```python
from build123d import *

# Parameters (mm, degrees)
SKETCH005_R       = 41.5
SKETCH005_R_2     = 12.75
PAD001_DEPTH      = 16.5
CYLINDER003_R     = 16
CYLINDER003_DEPTH = 25.2
CYLINDER008_R     = 4
CYLINDER008_DEPTH = 25
CYLINDER009_R     = 4
CYLINDER009_DEPTH = 25
POCKET_START      = -1.25
SKETCH084_R       = 48
SKETCH084_R_2     = 40
POCKET_DEPTH      = 14


with BuildPart() as part:
    # Sketch005 → Pad001 (new body)
    with BuildSketch(Plane.XY):
        with Locations((0, -21.25)):
            Circle(SKETCH005_R)
        Circle(SKETCH005_R_2, mode=Mode.SUBTRACT)
        with BuildLine():
            ThreePointArc((-31.480397, -26.993223), (-24.225688, -42.15732), (-10.285714, -51.551882))
            ThreePointArc((-10.285714, -51.551882), (-6.670071, -51.015521), (-5, -47.764147))
            Line((-5, -27.568098), (-5, -47.764147))
            ThreePointArc((-5, -27.568098), (-5.762291, -25.219217), (-7.758621, -23.765601))
            ThreePointArc((-16.637158, -18.660251), (-12.462129, -21.672456), (-7.758621, -23.765601))
            ThreePointArc((-16.637158, -18.660251), (-27.032318, -17.53007), (-31.480397, -26.993223))
        make_face(mode=Mode.SUBTRACT)
        with BuildLine():
            ThreePointArc((10.285714, -51.551882), (24.225688, -42.15732), (31.480397, -26.993223))
            ThreePointArc((31.480397, -26.993223), (27.032318, -17.53007), (16.637158, -18.660251))
            ThreePointArc((7.758621, -23.765601), (12.462129, -21.672456), (16.637158, -18.660251))
            ThreePointArc((7.758621, -23.765601), (5.762291, -25.219217), (5, -27.568098))
            Line((5, -27.568098), (5, -47.764147))
            ThreePointArc((5, -47.764147), (6.670071, -51.015521), (10.285714, -51.551882))
        make_face(mode=Mode.SUBTRACT)
    extrude(amount=-PAD001_DEPTH)

    # Cylinder003 → Cylinder003 (cut)
    with BuildSketch(Plane.XY.offset(-12.5)):
        Circle(CYLINDER003_R)
    extrude(amount=CYLINDER003_DEPTH, mode=Mode.SUBTRACT)

    # Cylinder008 → Cylinder008 (cut)
    with BuildSketch(Plane(origin=(23, 0, -13), x_dir=(1, 0, 0), z_dir=(0, 0, 1))):
        Circle(CYLINDER008_R)
    extrude(amount=CYLINDER008_DEPTH, mode=Mode.SUBTRACT)

    # Cylinder009 → Cylinder009 (cut)
    with BuildSketch(Plane(origin=(-23, 0, -13), x_dir=(1, 0, 0), z_dir=(0, 0, 1))):
        Circle(CYLINDER009_R)
    extrude(amount=CYLINDER009_DEPTH, mode=Mode.SUBTRACT)

    # Sketch084 → Pocket (cut)
    with BuildSketch(Plane.XY.offset(POCKET_START)):
        with Locations((0, -21.25)):
            Circle(SKETCH084_R)
        with Locations((0, -21.25)):
            Circle(SKETCH084_R_2, mode=Mode.SUBTRACT)
    extrude(amount=-POCKET_DEPTH, mode=Mode.SUBTRACT)


solid = part.part
```
The model under review builds one solid part; all positions refer to its coordinate system, in mm. A direction names the side the tool comes from. Round coordinates to 2 decimals unless told otherwise and drop trailing zeros. Loops run counter-clockwise (first coordinate to the right, second up) from the corner with the lowest first, then second, coordinate; pieces in that order, holes last. Notation, with made-up numbers: M 1,60.5 L 23,60.5 A21 ccw 23,69.5 Z; hole C 9,11 d7. An arc over 180 degrees is marked long. Put each result on its own line as item: value.
Q1. Consider section C-C, the plane y = 0. Give the boundary of the cut face in (x, z).
Result set:
outline: M -35.65,-16.5 L -12.75,-16.5 L -12.75,-12.5 L -16,-12.5 L -16,0 L -19,0 L -19,-13 L -27,-13 L -27,0 L -35.65,0 L -35.65,-1.25 L -33.89,-1.25 L -33.89,-15.25 L -35.65,-15.25 Z; M 12.75,-16.5 L 35.65,-16.5 L 35.65,-15.25 L 33.89,-15.25 L 33.89,-1.25 L 35.65,-1.25 L 35.65,0 L 27,0 L 27,-13 L 19,-13 L 19,0 L 16,0 L 16,-12.5 L 12.75,-12.5 Z
Q2. Consider section D-D, the plane y = -21.25. Give the boundary of the cut face in (x, z).
Result set:
outline: M -41.5,-16.5 L -30.62,-16.5 L -30.62,0 L -41.5,0 L -41.5,-1.25 L -40,-1.25 L -40,-15.25 L -41.5,-15.25 Z; M -13.17,-16.5 L 13.17,-16.5 L 13.17,0 L -13.17,0 Z; M 30.62,-16.5 L 41.5,-16.5 L 41.5,-15.25 L 40,-15.25 L 40,-1.25 L 41.5,-1.25 L 41.5,0 L 30.62,0 Z
Q3. Mouldability with a two-part tool opening along Y and no side actions: class faces 1 (the flat face through (5, -38, -8)), 2 (the cylindrical face through (-30.587, 6.798, -0.616)), 3 (the flat face through (-22, 13, -1.25)) as released by +Y, released by -Y, zero draft, split by the parting line, or undercut.
Result set:
face 1: undercut
face 2: split by the parting line
face 3: zero draft
Q4. Machinability: for faces 4 (the cylindrical face through (12.4, -21.71, -8.13)), 5 (the flat face through (23, 0, -13)), 6 (the flat face through (-22, 13, -15.25)), which of the approach directions +Z, -Z, +X, -X, +Y, -Y give a long, thin tool a straight path to every point of the face, cutting with its end or side? Answer none if there is none.
Result set:
face 4: +Z, -Z
face 5: +Z
face 6: none
Q5. For pin 1 (1.5 mm diameter, centred on x = 1.5, y = -36, fed in from +Z); pin 2 (9.5 mm diameter, centred on x = -2.5, y = 2.5, fed in from +Z); pin 3 (4 mm diameter, centred on y = -35, z = -8, fed in from +X); pin 4 (4 mm diameter, centred on x = 22.5, y = 1, fed in from +Z), all flat-tipped, find the tip position at first contact; note any pin that passes through.
Result set:
pin 1: stops at z = 0
pin 2: passes through
pin 3: stops at x = 38.24
pin 4: stops at z = -13
Q6. Consider section B-B, the plane z = -3. Give the boundary of the cut face in (x, y).
Result set:
outline: C 0,-21.25 d80; hole M -31.48,-26.99 A32 ccw -10.29,-51.55 A4 ccw -5,-47.76 L -5,-27.57 A4 ccw -7.76,-23.77 A25 cw -16.64,-18.66 A9 ccw Z; hole C -23,0 d8; hole C 0,0 d32; hole M 5,-47.76 A4 ccw 10.29,-51.55 A32 ccw 31.48,-26.99 A9 ccw 16.64,-18.66 A25 cw 7.76,-23.77 A4 ccw 5,-27.57 Z; hole C 23,0 d8
Q7. Consider section A-A, the plane x = 0. Give the boundary of the cut face in (y, z).
Result set:
outline: M -62.75,-16.5 L -12.75,-16.5 L -12.75,-12.5 L -16,-12.5 L -16,0 L -62.75,0 L -62.75,-1.25 L -61.25,-1.25 L -61.25,-15.25 L -62.75,-15.25 Z; M 12.75,-16.5 L 20.25,-16.5 L 20.25,-15.25 L 18.75,-15.25 L 18.75,-1.25 L 20.25,-1.25 L 20.25,0 L 16,0 L 16,-12.5 L 12.75,-12.5 Z
Q8. To check wall thickness, follow L1, parallel to Y at x = -8, z = -9.5; L2, parallel to Y at x = 0, z = -15.5; L3, parallel to Y at x = 0, z = -13.75. State the ranges of each line that lie inside material, in increasing order.
Result set:
L1: y = -60.44 to -51.64, -23.69 to -13.86, 13.86 to 17.94
L2: y = -62.75 to -12.75, 12.75 to 20.25
L3: y = -61.25 to -12.75, 12.75 to 18.75
